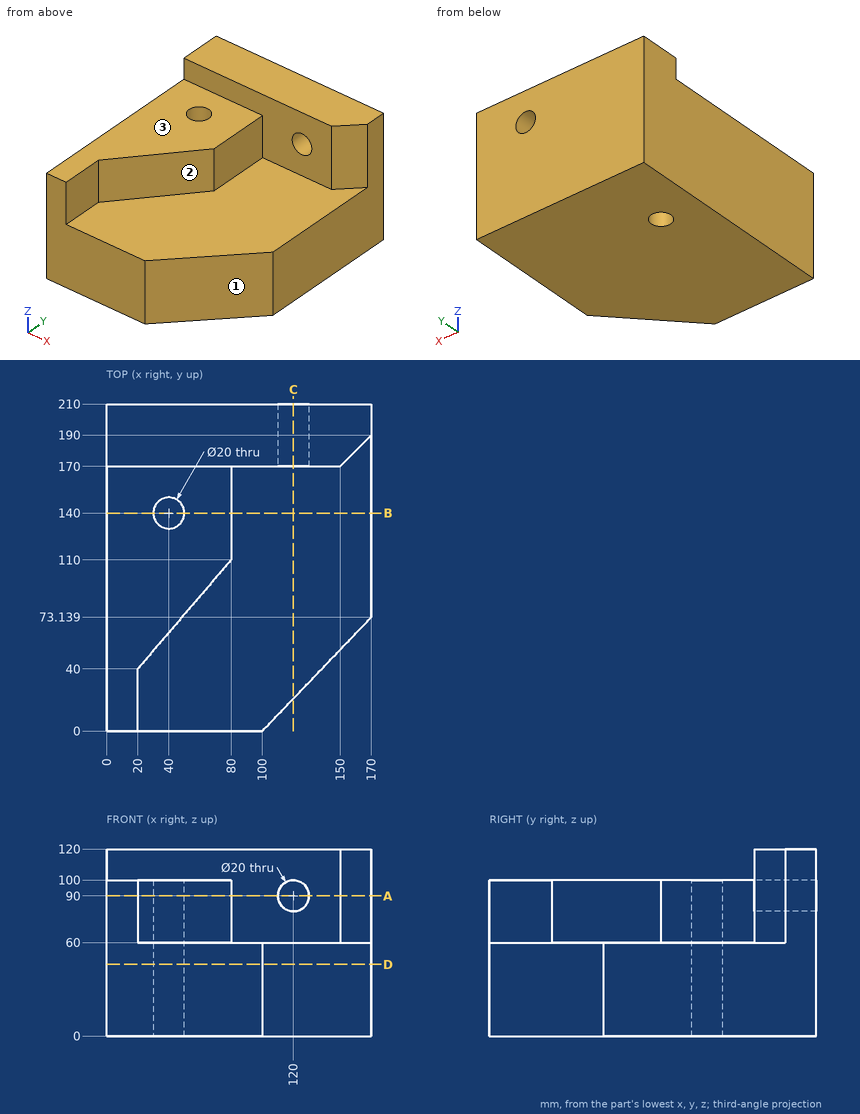
For this review, use the dimensioned drawing (mm, ordinates from the lowest corner) and the shaded views. A direction names the side the tool comes from. Round coordinates to 2 decimals unless told otherwise and drop trailing zeros. Write each loop counter-clockwise with the first axis right and the second up, starting at its lowest first coordinate (ties: lowest second). Pieces come first, ordered by that corner, then holes. Notation, with made-up numbers: (-33, -33) -> (-5, -33) arc R16 cw to (-5, -18) -> close; hole circle Ø11 at (70.25, 78.25). An arc over 180 degrees is marked (long way). One line per item, written item: value. Start each with the question number.
Q1. To check wall thickness, follow probe 1 along Y at (x, z) = (40, 46); probe 2 along X at (y, z) = (202.5, 90); probe 3 along X at (y, z) = (140, 34.5). State the ranges of each line that lie inside material, in increasing order.
Q2. Add section C-C (x = 120). Give the boundary of the cut face in (y, z), then the cut area to 3 significant figures.
Q3. Add section A-A (z = 90). Give the boundary of the cut face in (x, y).
Q4. Add section B-B (y = 140). Give the boundary of the cut face in (x, z).
Q5. Add section D-D (z = 46). Give the boundary of the cut face in (x, y), then the cut area to 3 significant figures.
Q6. Insertion check: P1, Ø6, axis at y = 58, z = 30, coming from the +X side; P2, Ø18, axis at x = 40, y = 140, coming from the +Z side; P3, Ø3, axis at x = 134.5, y = 141, coming from the +Z side. Each pin has a flat end and moves straight along its axis. Give the tip position at first contact, or say it passes through.
Q7. Tool access review of the marked faces 1, 2 and 3: name each direction out of +Z, -Z, +X, -X, +Y, -Y from which nothing blocks a thin tool from reaching the whole face with its end or side.
Response:
1. probe 1: y = 0 to 130, 150 to 210
1. probe 2: x = 0 to 110, 130 to 170
1. probe 3: x = 0 to 30, 50 to 170
2. outline: (20.9, 0) -> (210, 0) -> (210, 80) -> (170, 80) -> (170, 60) -> (20.9, 60) -> close; (170, 100) -> (210, 100) -> (210, 120) -> (170, 120) -> close
2. area: 12,900 mm^2
3. outline: (0, 0) -> (20, 0) -> (20, 40) -> (80, 110) -> (80, 170) -> (110, 170) -> (110, 210) -> (0, 210) -> close; (130, 170) -> (150, 170) -> (170, 190) -> (170, 210) -> (130, 210) -> close; hole circle Ø20 at (40, 140)
4. outline: (0, 0) -> (30, 0) -> (30, 100) -> (0, 100) -> close; (50, 0) -> (170, 0) -> (170, 60) -> (80, 60) -> (80, 100) -> (50, 100) -> close
5. outline: (0, 0) -> (100, 0) -> (170, 73.14) -> (170, 210) -> (0, 210) -> close; hole circle Ø20 at (40, 140)
5. area: 32,800 mm^2
6. P1: stops at x = 158.38
6. P2: passes through
6. P3: stops at z = 60
7. face 1: +Z, -Z, +X, -Y
7. face 2: +Z, +X, -Y
7. face 3: +Z, +X, -X, -Y
